Source: CAD feature listing. Evaluate the final solid. Frame: model axes, mm. A direction names the side the tool comes from. Give positions to 0.01 mm unless a question says otherwise; leave off trailing zeros. Order: outer loops, then holes, each group sorted by start corner. A loop starts at its lowest first (then second) coordinate and runs counter-clockwise, first axis right, second up.
Autodesk Inventor part; units mm, degrees
ref_plane "YZ Plane" through (0, 0, 0) normal (1, 0, 0) x (0, 1, 0)
ref_plane "XZ Plane" through (0, 0, 0) normal (0, 1, 0) x (-1, 0, 0)
ref_plane "XY Plane" through (0, 0, 0) normal (0, 0, 1) x (1, 0, 0)
sketch "Sketch1" plane through (0, 0, 0) normal (0, 0, 1) x (1, 0, 0)
  line L0 (-50, -50) -> (0, 0)
  line L1 (125, 0) -> (0, 0)
  line L2 (125, 0) -> (175, -50)
  line L3 (178, -50) -> (175, -50)
  line L4 (-53, -50) -> (-50, -50)
  circle A0 centre (117.5, -37.5) radius 1.5
  arc A1 (114.25, -43.8002) -> (114.25, -56.1998) centre (117.5, -50) ccw
  arc A2 (120.75, -56.1998) -> (120.75, -43.8002) centre (117.5, -50) ccw
  line L5 (-53, -50) -> (0, 3)
  line L6 (0, 3) -> (125, 3)
  line L7 (125, 3) -> (178, -50)
extrude "Extrusion1" add sketch "Sketch1" along normal blind 53 contours L4 L5 L6 L7 L3 L2 L1 L0
sketch "Sketch2" plane through (0, 3, 0) normal (0, 1, 0) x (1, 0, 0)
  line L0 (0, -43) -> (125, -43)
  line L1 (125, -53) -> (0, -53)
  circle A0 centre (31.25, -48) radius 1.8
  circle A1 centre (93.75, -48) radius 1.8
  line L2 (-53, -10.625) -> (-53, -53)
  line L3 (-53, -53) -> (-50, -53)
  line L4 (-50, -53) -> (0, -53)
  line L5 (0, 0) -> (-53, 0)
  line L6 (-53, 0) -> (-53, -53)
  line L7 (0, -53) -> (-53, -53)
  line L8 (0, 0) -> (0, -53)
  circle A2 centre (31.25, -48) radius 1.6
  circle A3 centre (93.75, -48) radius 1.6
  dimension "d2" = 3.2
  dimension "d3" = 3.2
extrude "Extrusion2" cut sketch "Sketch2" against normal up to surface (3 mm away) contours A0 | A1 | A2 | A3
sketch "Sketch3" plane through (0, 0, 0) normal (0, 0, -1) x (-1, 0, 0)
  line L0 (0, 3) -> (53, -50)
  line L1 (-125, 3) -> (0, 3)
  line L2 (-178, -50) -> (-125, 3)
  line L3 (-175, -50) -> (-178, -50)
  line L4 (-125, 0) -> (-175, -50)
  line L5 (0, 0) -> (-125, 0)
  line L6 (50, -50) -> (0, 0)
  line L7 (53, -50) -> (43, -40)
  line L8 (43, -40) -> (40, -40)
  line L9 (40, -40) -> (50, -50)
  line L10 (50, -50) -> (53, -50)
  line L11 (53, -50) -> (50, -50)
extrude "Extrusion3" cut sketch "Sketch3" against normal blind 34.125
chamfer "Chamfer2" distance 10 angle 45 1 edges at (-51.5, -50, 34.125)
properties part number "obudowa_górna_krótka" material "ABS Plastic"
1) Section query A-A, the plane y = -8.5. Return the cut outline in (x, z) (3 decimals).
Report:
outline: (-11.5, 34.125) - (-8.5, 34.125) - (-8.5, 53) - (-11.5, 53) - close; (133.5, 34.125) - (136.5, 34.125) - (136.5, 53) - (133.5, 53) - close
2) Section query B-B, the plane z = 40. Return the cut outline in (x, y) (3 decimals).
Report:
outline: (-48.875, -45.875) - (-45.875, -45.875) - (0, 0) - (125, 0) - (175, -50) - (178, -50) - (125, 3) - (0, 3) - close
3) Pin query (flat end, axial travel): pin 1 (10 mm diameter, centred on y = -16.5, z = 45.5, fed in from -X); pin 2 (8 mm diameter, centred on x = 129.5, z = 50, fed in from +Y); pin 3 (5.5 mm diameter, centred on x = 35.5, z = 40.5, fed in from -Y); pin 4 (2 mm diameter, centred on x = 31.25, z = 48, fed in from +Y). Return the tip coordinate at first contact, or that it passes through.
Report:
pin 1: stops at x = -24.5
pin 2: stops at y = 2.5
pin 3: stops at y = 0
pin 4: passes through
4) Material intervals for L1, parallel to X at y = 1.7, z = 48; L2, parallel to Z at x = 31.25, y = 1.15 (3 decimals); L3, parallel to X at y = 0.75, z = 48, sorted ascending.
Report:
L1: x = -1.3 to 29.45, 33.05 to 91.95, 95.55 to 126.3
L2: z = 34.125 to 46.2, 49.8 to 53
L3: x = -2.25 to 29.45, 33.05 to 91.95, 95.55 to 127.25
5) Reachability of faces 1 (the flat face through (150, -25, 43)), 2 (the flat face through (-27, -24, 43)), 3 (the flat face through (-46.47, -45.023, 39.148)) from +Z, -Z, +X, -X, +Y, -Y: full face, straight path, thin tool, end or side. Return the list, or none.
Report:
face 1: +Z, -Z, -Y
face 2: +Z, -Z, -X, +Y
face 3: -Z, -X, -Y
6) Draft query along X for faces 4 (the flat face through (62, 3, 43)), 5 (the flat face through (63, 0, 43)), 6 (the flat face through (151, -23, 43)). Return one class per face: +X half, -X half, draft (parallel to the pull), parting line (faces both ways), or undercut.
Report:
face 4: draft
face 5: undercut
face 6: +X half
7) Section query C-C, the plane x = 81.5. Return the cut outline in (y, z) (3 decimals), and give its area (3 significant figures).
Report:
outline: (0, 34.125) - (3, 34.125) - (3, 53) - (0, 53) - close
area: 56.6 mm2
